Source: CAD feature listing. Evaluate the final solid. Frame: model axes, mm. Face numbers are marked on the shaded views. A direction names the side the tool comes from. Round coordinates to 2 decimals unless told otherwise and drop trailing zeros. Loops run counter-clockwise (first coordinate to the right, second up) from the corner with the lowest first, then second, coordinate; pieces in that order, holes last.
Item 1: Section query D-D on y = 7.25. Return loops of the section in (x, z) (3 decimals), then the cut area to 3 significant figures.
Item 2: Access query for the marked faces 4 and 5. Directions: +Z, -Z, +X, -X, +Y, -Y. A direction counts if a zero-diameter tool reaches every point of the face in a straight line with its end or side. Return the directions, or none.
Item 3: Section query C-C on y = 1.25. Return loops of the section in (x, z).
Item 4: Ray query, L1, parallel to X at y = 4.75, z = 0; L2, parallel to Y at x = 4.5, z = -1.5 (3 decimals); L3, parallel to Z at x = 1, y = 5.75. Return the intervals inside material, ascending.
Item 5: First-contact query: P1, Ø2, axis at x = -2.5, z = 4.5, coming from the -Y side; P2, Ø2, axis at y = 2, z = 1, coming from the -X side. Flat tips, straight axial feed; report the tip coordinate or a pass-through.
Item 6: Section query A-A on x = 0. Return loops of the section in (y, z) (3 decimals).
Item 7: Section query B-B on z = 0. Return loops of the section in (x, y) (3 decimals).
Item 8: Pull-direction query (X, two-part tool) for the marked faces 1, 2 and 3; classes: released by +X, released by -X, zero draft, split by the parting line, or undercut.
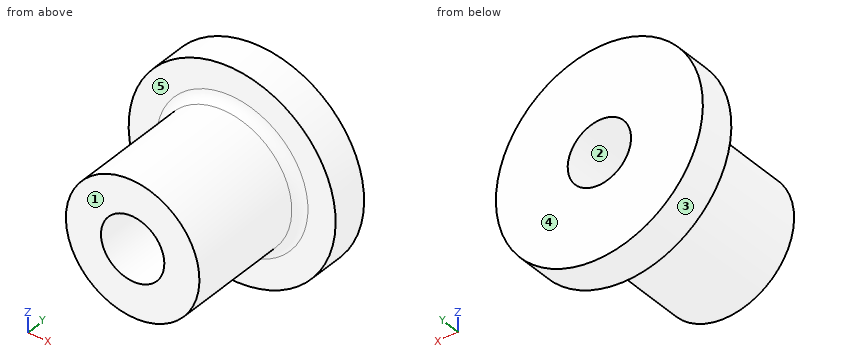
```python
from build123d import *

# Parameters (mm, degrees)
SKETCH1_R           = 3.687
SKETCH1_R_2         = 1.75
BOSS_EXTRUDE1_DEPTH = 6.985
SKETCH2_R           = 5.715
SKETCH2_R_2         = 1.75
BOSS_EXTRUDE2_DEPTH = 2
FILLET1_R           = 0.5


with BuildPart() as part:
    # Sketch1 → Boss-Extrude1 (new body)
    with BuildSketch(Plane(origin=(0, 0, 0), x_dir=(1, 0, 0), z_dir=(0, 1, 0))):
        with Locations(Location((0, 0, 0), (0, 0, 270))):
            Circle(SKETCH1_R)
        with Locations(Location((0, 0, 0), (0, 0, 270))):
            Circle(SKETCH1_R_2, mode=Mode.SUBTRACT)
    extrude(amount=BOSS_EXTRUDE1_DEPTH)

    # Sketch2 → Boss-Extrude2 (add)
    with BuildSketch(Plane(origin=(0, 6.985, 0), x_dir=(1, 0, 0), z_dir=(0, 1, 0))):
        with Locations(Location((0, 0, 0), (0, 0, 270))):
            Circle(SKETCH2_R)
        with Locations(Location((0, 0, 0), (0, 0, 270))):
            Circle(SKETCH2_R_2, mode=Mode.SUBTRACT)
    extrude(amount=BOSS_EXTRUDE2_DEPTH)

    # Fillet1
    fillet1_edges = [part.edges().sort_by_distance(p)[0] for p in [
        (0, 6.985, -3.687),
    ]]
    fillet(fillet1_edges, radius=FILLET1_R)


solid = part.part
```
Data:
1. outline: circle Ø11.43 at (0, 0); hole circle Ø3.5 at (0, 0)
1. area: 93.0 mm2
2. face 4: +Z, -Z, +X, -X, +Y
2. face 5: -Y
3. outline: circle Ø7.37 at (0, 0); hole circle Ø3.5 at (0, 0)
4. L1: x = -3.69 to -1.75, 1.75 to 3.69
4. L2: y = 6.985 to 8.985
4. L3: z = -3.55 to -1.44, 1.44 to 3.55
5. P1: stops at y = 6.98
5. P2: stops at x = -3.69
6. outline: (0, -3.687) - (6.485, -3.687) arc R0.5 cw to (6.985, -4.187) - (6.985, -5.715) - (8.985, -5.715) - (8.985, -1.75) - (0, -1.75) - close; (0, 1.75) - (8.985, 1.75) - (8.985, 5.715) - (6.985, 5.715) - (6.985, 4.187) arc R0.5 cw to (6.485, 3.687) - (0, 3.687) - close
7. outline: (-5.715, 6.985) - (-4.187, 6.985) arc R0.5 cw to (-3.687, 6.485) - (-3.687, 0) - (-1.75, 0) - (-1.75, 8.985) - (-5.715, 8.985) - close; (1.75, 0) - (3.687, 0) - (3.687, 6.485) arc R0.5 cw to (4.187, 6.985) - (5.715, 6.985) - (5.715, 8.985) - (1.75, 8.985) - close
8. face 1: zero draft
8. face 2: undercut
8. face 3: split by the parting line
